For this review, take the finished solid that the model builds, in its own axes (mm). A direction names the side the tool comes from. Coordinates: 2 decimals unless noted, no trailing zeros. Loops run counter-clockwise (first coordinate to the right, second up) from the corner with the lowest first, then second, coordinate; pieces in that order, holes last. Notation, with made-up numbers: (69.5, -36.5) -> (98.5, -36.5) arc R21 cw to (98.5, -18.5) -> close; hole circle Ø3 at (-33.5, 52). An arc over 180 degrees is marked (long way). Answer in a Markdown table with one row per item.
from build123d import *

# Parameters (mm, degrees)
BOSS_EXTRUDE1_DEPTH = 3
SKETCH2_W           = 10
SKETCH2_H           = 5
CUT_EXTRUDE1_DEPTH  = 3


with BuildPart() as part:
    # Sketch1 → Boss-Extrude1 (new body)
    with BuildSketch(Plane.XY):
        with BuildLine():
            Line((-5, 0), (-5, -3))
            Line((-5, -3), (0, -3))
            Line((0, -3), (0, -113.008152331))
            Line((0, -113.008152331), (-5, -113.008152331))
            Line((-5, -113.008152331), (-5, -116))
            Line((-5, -116), (-25, -116))
            Line((-25, -116), (-25, -113))
            Line((-25, -113), (-30, -113))
            Line((-30, -113), (-30, -88.243527021))
            ThreePointArc((-30, -88.243527021), (-4.280708477, -60.801240722), (-30, -33.358954423))
            Line((-30, -33.358954423), (-30, -3))
            Line((-30, -3), (-25, -3))
            Line((-25, -3), (-25, 0))
            Line((-25, 0), (-5, 0))
        make_face()
    extrude(amount=BOSS_EXTRUDE1_DEPTH)

    # Sketch2 → Cut-Extrude1 (cut)
    with BuildSketch(Plane.XY.offset(3)):
        with Locations((-25, -107.5)):
            Rectangle(SKETCH2_W, SKETCH2_H)
        with Locations((-25, -13.5)):
            Rectangle(SKETCH2_W, SKETCH2_H)
    extrude(amount=-CUT_EXTRUDE1_DEPTH, mode=Mode.SUBTRACT)


solid = part.part
Item 1: For L1, parallel to Y at x = -20.25, z = 2; L2, parallel to Y at x = -6.5, z = 1.25; L3, parallel to Y at x = -19, z = 0.4, list the stretches that pass through material, from the lowest coordinate up.
Worked answers:
| item | result |
|---|---|
| L1 | -116 to -110, -105 to -85.77, -35.84 to -16, -11 to 0 |
| L2 | -116 to -71.62, -49.98 to 0 |
| L3 | -116 to -85.15, -36.45 to 0 |
Item 2: The part is to be moulded in two halves that separate along Y. For faces 1 (the flat face through (-30, -97, 1)), 2 (the flat face through (-2, -113.008, 1)), 3 (the flat face through (-20, -108, 2)), say which applies: +Y half, -Y half, draft (parallel to the pull), parting line (faces both ways), or undercut.
Worked answers:
| item | result |
|---|---|
| face 1 | draft |
| face 2 | -Y half |
| face 3 | undercut |
Item 3: Take a section at D-D, the plane y = -12. State the section outline as (x, z) points, and give its area (3 significant figures).
Worked answers:
| item | result |
|---|---|
| outline | (-20, 0) -> (0, 0) -> (0, 3) -> (-20, 3) -> close |
| area | 60.0 mm² |
Item 4: Take a section at B-B, the plane x = -24. State the section outline as (y, z) points.
Worked answers:
| item | result |
|---|---|
| outline | (-116, 0) -> (-110, 0) -> (-110, 3) -> (-116, 3) -> close; (-105, 0) -> (-87.18, 0) -> (-87.18, 3) -> (-105, 3) -> close; (-34.42, 0) -> (-16, 0) -> (-16, 3) -> (-34.42, 3) -> close; (-11, 0) -> (0, 0) -> (0, 3) -> (-11, 3) -> close |
Item 5: Insertion check: pin 1 (0.9 mm diameter, centred on y = -13, z = 2, fed in from -X); pin 2 (0.9 mm diameter, centred on x = -2.5, z = 2, fed in from +Y); pin 3 (1.5 mm diameter, centred on x = -27, z = 2, fed in from -Y). Each pin has a flat end and moves straight along its axis. Give the tip position at first contact, or say it passes through.
Worked answers:
| item | result |
|---|---|
| pin 1 | x = -20 |
| pin 2 | y = -3 |
| pin 3 | y = -113 |
Item 6: For faces 4 (the flat face through (-25, -2, 1)), 5 (the flat face through (-5, -114, 1)), 6 (the flat face through (-25, -110, 2)), list the 3-axis set-ups (+Z, -Z, +X, -X, +Y, -Y) from which the entire face can be reached by the end or side of a thin tool; tool diameter is ignored.
Worked answers:
| item | result |
|---|---|
| face 4 | +Z, -Z, -X, +Y |
| face 5 | +Z, -Z, +X, -Y |
| face 6 | +Z, -Z, -X |
Item 7: Take a section at A-A, the plane x = -17. State the section outline as (y, z) points, and give its area (3 significant figures).
Worked answers:
| item | result |
|---|---|
| outline | (-116, 0) -> (-83.99, 0) -> (-83.99, 3) -> (-116, 3) -> close; (-37.61, 0) -> (0, 0) -> (0, 3) -> (-37.61, 3) -> close |
| area | 209 mm² |
Item 8: Take a section at C-C, the plane z = 2.4. State the section outline as (x, y) points, and give its area (3 significant figures).
Worked answers:
| item | result |
|---|---|
| outline | (-30, -113) -> (-25, -113) -> (-25, -116) -> (-5, -116) -> (-5, -113.01) -> (0, -113.01) -> (0, -3) -> (-5, -3) -> (-5, 0) -> (-25, 0) -> (-25, -3) -> (-30, -3) -> (-30, -11) -> (-20, -11) -> (-20, -16) -> (-30, -16) -> (-30, -33.36) arc R27.5 cw to (-30, -88.24) -> (-30, -105) -> (-20, -105) -> (-20, -110) -> (-30, -110) -> close |
| area | 2,230 mm² |
